The model under review builds one solid part; all positions refer to its coordinate system, in mm. A direction names the side the tool comes from. Coordinates: 2 decimals unless noted, no trailing zeros. Order: outer loops, then holes, each group sorted by start corner. A loop starts at its lowest first (then second) coordinate and runs counter-clockwise, first axis right, second up. Notation, with made-up numbers: (48.5, -17) -> (96.5, -17) arc R21 cw to (96.5, 7) -> close; hole circle Ø3 at (-38.5, 6.25). An arc over 180 degrees is marked (long way). Put each result on its own line as item: value.
from build123d import *
from build123d.topology import SkipClean

# Parameters (mm, degrees)
SKETCH1_R               = 25
SKETCH1_R_2             = 20.15
BOSS_EXTRUDE1_DEPTH     = 10
BOSS_EXTRUDE2_START     = 5
SKETCH2_R               = 25
SKETCH2_R_2             = 1.375
SKETCH2_R_3             = 5
BOSS_EXTRUDE2_DEPTH     = 5
SKETCH3_R               = 3
CUT_EXTRUDE1_DEPTH      = 2
CUT_EXTRUDE2_DEPTH      = 38
CUT_EXTRUDE2_DEPTH_BACK = 33
SKETCH4_R               = 1.625
SKETCH5_R               = 21.025
CUT_EXTRUDE3_DEPTH      = 10
SKETCH6_R               = 25
SKETCH6_R_2             = 21.025
BOSS_EXTRUDE3_DEPTH     = 5
FILLET1_R               = 2


with BuildPart() as part:
    # Sketch1 → Boss-Extrude1 (new body)
    with BuildSketch(Plane.XY):
        Circle(SKETCH1_R)
        Circle(SKETCH1_R_2, mode=Mode.SUBTRACT)
    extrude(amount=BOSS_EXTRUDE1_DEPTH)

    # Sketch2 → Boss-Extrude2 (add)
    with BuildSketch(Plane(origin=(0, 0, 0), x_dir=(-1, 0, 0), z_dir=(0, 0, -1)).offset(BOSS_EXTRUDE2_START)):
        Circle(SKETCH2_R)
        with Locations((-11, 0)):
            Circle(SKETCH2_R_2, mode=Mode.SUBTRACT)
        with Locations((-7.778174593, 7.778174593)):
            Circle(SKETCH2_R_2, mode=Mode.SUBTRACT)
        with Locations((0, 11)):
            Circle(SKETCH2_R_2, mode=Mode.SUBTRACT)
        with Locations((7.778174593, 7.778174593)):
            Circle(SKETCH2_R_2, mode=Mode.SUBTRACT)
        with Locations((11, 0)):
            Circle(SKETCH2_R_2, mode=Mode.SUBTRACT)
        with Locations((7.778174593, -7.778174593)):
            Circle(SKETCH2_R_2, mode=Mode.SUBTRACT)
        with Locations((0, -11)):
            Circle(SKETCH2_R_2, mode=Mode.SUBTRACT)
        with Locations((-7.778174593, -7.778174593)):
            Circle(SKETCH2_R_2, mode=Mode.SUBTRACT)
        Circle(SKETCH2_R_3, mode=Mode.SUBTRACT)
    extrude(amount=-BOSS_EXTRUDE2_DEPTH)

    # Sketch3 → Cut-Extrude1 (cut)
    with BuildSketch(Plane.XY):
        with Locations((0, 11)):
            Circle(SKETCH3_R)
        with Locations((7.778174593, 7.778174593)):
            Circle(SKETCH3_R)
        with Locations((11, 0)):
            Circle(SKETCH3_R)
        with Locations((7.778174593, -7.778174593)):
            Circle(SKETCH3_R)
        with Locations((0, -11)):
            Circle(SKETCH3_R)
        with Locations((-7.778174593, -7.778174593)):
            Circle(SKETCH3_R)
        with Locations((-11, 0)):
            Circle(SKETCH3_R)
        with Locations((-7.778174593, 7.778174593)):
            Circle(SKETCH3_R)
    extrude(amount=-CUT_EXTRUDE1_DEPTH, mode=Mode.SUBTRACT)

    # Sketch4 → Cut-Extrude2 (cut, two sides: drawn at the far end of the back side and taken through both)
    with BuildSketch(Plane(origin=(0, 0, 0), x_dir=(1, 0, 0), z_dir=(0, 1, 0)).offset(-CUT_EXTRUDE2_DEPTH_BACK)):
        with Locations(Location((0, -5, 0), (0, 0, 90))):
            Circle(SKETCH4_R)
    extrude(amount=CUT_EXTRUDE2_DEPTH + CUT_EXTRUDE2_DEPTH_BACK, mode=Mode.SUBTRACT)

    # Sketch5 → Cut-Extrude3 (cut)
    with BuildSketch(Plane.XY.offset(10)):
        Circle(SKETCH5_R)
    extrude(amount=-CUT_EXTRUDE3_DEPTH, mode=Mode.SUBTRACT)

    # Sketch6 → Boss-Extrude3 (add)
    with SkipClean():  # the faces are left unmerged after this step: merging them gives an invalid solid
        with BuildSketch(Plane.XY.offset(10)):
            with Locations(Location((0, 0, 0), (0, 0, 180))):
                Circle(SKETCH6_R)
            Circle(SKETCH6_R_2, mode=Mode.SUBTRACT)
        extrude(amount=BOSS_EXTRUDE3_DEPTH)

    # Fillet1
    fillet1_edges = [part.edges().sort_by_distance(p)[0] for p in [
        (-21.025, 0, 15),
    ]]
    fillet(fillet1_edges, radius=FILLET1_R)


solid = part.part
Item 1: Mouldability with a two-part tool opening along X and no side actions: class faces 1 (the flat face through (0.3, -5.2, -5)), 2 (the flat face through (-6, -8, -2)) as +X half, -X half, draft (parallel to the pull), parting line (faces both ways), or undercut.
Answers below:
face 1: draft
face 2: undercut
Item 2: Consider section B-B on z = 5. Write out the cut boundary in (x, y) (3 decimals).
Answers below:
outline: (-1.625, -24.947) -> (-1.625, -20.962) arc R21.025 cw to (-1.625, 20.962) -> (-1.625, 24.947) arc R25 ccw to start; (1.625, -24.947) arc R25 ccw to (1.625, 24.947) -> (1.625, 20.962) arc R21.025 cw to (1.625, -20.962) -> close
Item 3: For faces 3 (the cylindrical face through (9.39, -5.25, -0.99)), 4 (the cylindrical face through (7.144, -8.998, -3.521)), list the 3-axis set-ups (+Z, -Z, +X, -X, +Y, -Y) from which the entire face can be reached by the end or side of a thin tool; tool diameter is ignored.
Answers below:
face 3: +Z
face 4: +Z, -Z
Item 4: Consider section A-A on y = 0. Count the separate pieces of the cut face and the enclosed holes in it, and give its area (3 significant figures).
Answers below:
separate pieces: 4
enclosed holes: 0
area: 277 mm^2
Item 5: For line 1 (Y direction, x = 0, z = -4.35) (3 decimals); line 2 (Z direction, x = -5, y = 13); line 3 (Z direction, x = 9, y = 1), list the stretches that pass through material, from the lowest coordinate up. Write a range as from..to.
Answers below:
line 1: -25..-12.375, -9.625..-5, 5..9.625, 12.375..25
line 2: -5..0
line 3: -5..-2
Item 6: For pin 1 Ø3 at (x, y) = (11, 18) entering from +Z; pin 2 Ø8 at (x, y) = (-17, -6.5) entering from +Z; pin 3 Ø5 at (x, y) = (7.78, -7.78) entering from +Z; pin 4 Ø3 at (x, y) = (7.78, -7.78) entering from -Z, all flat-tipped, find the tip position at first contact; note any pin that passes through.
Answers below:
pin 1: z = 14.95
pin 2: z = 14.82
pin 3: z = -2
pin 4: z = -5
Item 7: Consider section D-D on z = 1.5. Write out the cut boundary in (x, y) (3 decimals).
Answers below:
outline: circle Ø50 at (0, 0); hole circle Ø42.05 at (0, 0)
